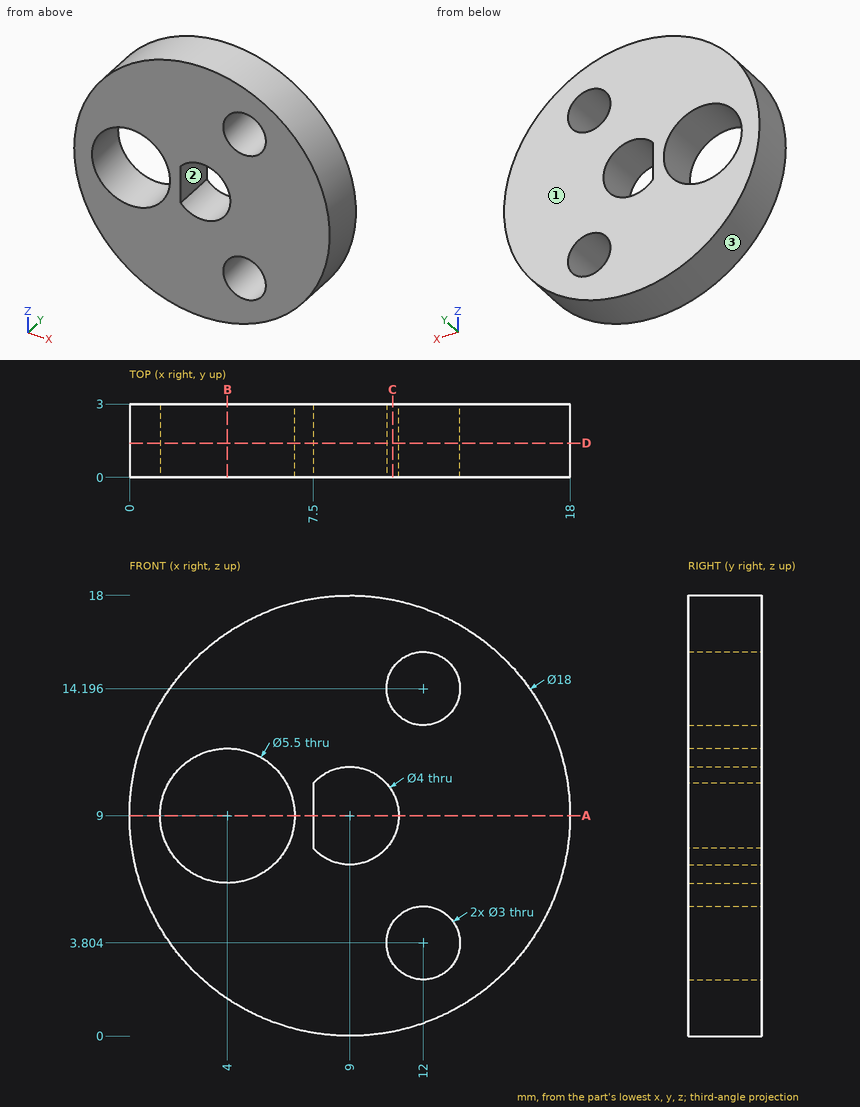
Study the drawing (mm; zero at the part's minimum x, y, z) and answer. Round coordinates to 2 decimals unless told otherwise and drop trailing zeros. Write each loop counter-clockwise with the first axis right and the second up, starting at its lowest first coordinate (ties: lowest second). Pieces come first, ordered by that corner, then holes.
1) A cutting plane is placed at D-D on y = 1.4. Determine the outline of the cut face in (x, z), and give its area (3 significant figures).
2) A cutting plane is placed at A-A on z = 9. Determine the outline of the cut face in (x, y).
3) A flat-ended cylindrical pin translates along its axis: P1, Ø1.5, axis at x = 10.5, y = 0.5, coming from the +Z side. Find the tip coordinate at first contact, or state that the pin passes through.
4) A cutting plane is placed at C-C on x = 10.75. Determine the outline of the cut face in (y, z) (1 decimal).
5) A cutting plane is placed at B-B on x = 4. Determine the outline of the cut face in (y, z).
6) Determine the mould class of the marked faces 1, 2 and 3 for opening direction Z: pulls with the +Z half, pulls with the -Z half, needs draft (parallel to the pull), parting line crosses it, or undercut.
7) Consider probe 1 along Z at (x, y) = (11.25, 1.25) (1 decimal); probe 2 along X at (y, z) = (2.1, 10.75); probe 3 along X at (y, z) = (2.65, 8) (1 decimal). Determine where each line is inside the solid, lowest interval first.
Entries:
1. outline: circle Ø18 at (9, 9); hole circle Ø5.5 at (4, 9); hole (7.5, 7.68) arc R2 ccw (long way) to (7.5, 10.32) - close; hole circle Ø3 at (12, 3.8); hole circle Ø3 at (12, 14.2)
1. area: 205 mm2
2. outline: (0, 0) - (1.25, 0) - (1.25, 3) - (0, 3) - close; (6.75, 0) - (7.5, 0) - (7.5, 3) - (6.75, 3) - close; (11, 0) - (18, 0) - (18, 3) - (11, 3) - close
3. P1: stops at z = 17.97
4. outline: (0, 0.2) - (3, 0.2) - (3, 3) - (0, 3) - close; (0, 4.6) - (3, 4.6) - (3, 8) - (0, 8) - close; (0, 10) - (3, 10) - (3, 13.4) - (0, 13.4) - close; (0, 15) - (3, 15) - (3, 17.8) - (0, 17.8) - close
5. outline: (0, 1.52) - (3, 1.52) - (3, 6.25) - (0, 6.25) - close; (0, 11.75) - (3, 11.75) - (3, 16.48) - (0, 16.48) - close
6. face 1: needs draft
6. face 2: undercut
6. face 3: parting line crosses it
7. probe 1: z = 0.3 to 2.5, 5.1 to 12.9, 15.5 to 17.7
7. probe 2: x = 0.17 to 1.88, 6.12 to 8.03, 9.97 to 17.83
7. probe 3: x = 0.1 to 1.4, 6.6 to 7.5, 10.7 to 17.9
